Geometry check sheet. Reference: the model listing, model coordinates, mm. Face numbers are marked on the shaded views. A direction names the side the tool comes from. Give positions to 0.01 mm unless a question says otherwise; leave off trailing zeros. Order: outer loops, then holes, each group sorted by start corner. A loop starts at its lowest first (then second) coordinate and runs counter-clockwise, first axis right, second up. Notation, with made-up numbers: M 21,-24.75 L 64,-24.75 A15 ccw 64,-11.75 Z; hole C 33,-8.75 d5. An arc over 180 degrees is marked long. One line per question, with ' | ' between items. Start each with the question number.
from build123d import *

# Parameters (mm, degrees)
SKETCH1_R           = 15
BOSS_EXTRUDE2_DEPTH = 60


with BuildPart() as part:
    # Sketch1 → Boss-Extrude2 (new body)
    # profile 1 of 2: a face of its own
    with BuildSketch(Plane.XY):
        with BuildLine():
            Line((-12.60240546, 38.711870299), (-12.60240546, -11.288129701))
            Line((-12.60240546, -11.288129701), (47.39759454, -11.288129701))
            Line((47.39759454, -11.288129701), (47.39759454, 38.711870299))
            ThreePointArc((47.39759454, 38.711870299), (17.39759454, 68.711870299), (-12.60240546, 38.711870299))
        make_face()
        with Locations((17.39759454, 38.711870299)):
            Circle(SKETCH1_R, mode=Mode.SUBTRACT)
    # profile 2 of 2: a face of its own
    with BuildSketch(Plane.XY):
        Polygon((-42.60240546, -11.288129701), (77.39759454, -11.288129701), (77.39759454, -36.288129701), (62.39759454, -36.288129701), (62.39759454, -21.288129701), (-27.60240546, -21.288129701), (-27.60240546, -36.288129701), (-42.60240546, -36.288129701), align=None)
    extrude(amount=BOSS_EXTRUDE2_DEPTH)


solid = part.part
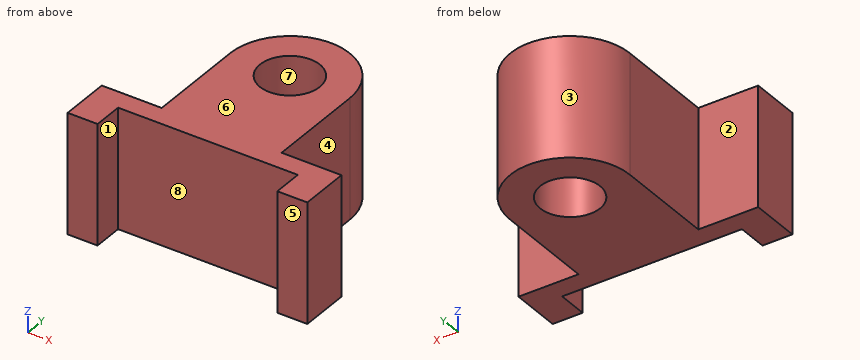
Item 1: Cross-section at C-C, the plane x = 4. Record the cut outline in (y, z).
Item 2: Depth check by flat-ended pin: pin 1 (25 mm diameter, centred on y = 20, z = 33, fed in from +X); pin 2 (18 mm diameter, centred on x = 4, z = 15.5, fed in from -Y); pin 3 (15 mm diameter, centred on y = 8, z = 20, fed in from -X); pin 4 (5 mm diameter, centred on x = 47.5, y = 18.5, fed in from +Z). Enter the tip coordinate at first touch or a pass-through.
Item 3: Cross-section at D-D, the plane x = -33. Record the cut outline in (y, z), plus the area to 3 significant figures.
Item 4: Material ranges on line 1 along X through (y, z) = (-32, 18.5); line 2 along Y through (x, z) = (70.5, 30); line 3 along Y through (x, z) = (-26.5, 45), recorded low to high.
Item 5: Cross-section at B-B, the plane z = 46.5. Record the cut outline in (x, y), plus the area to 3 significant figures.
Item 6: Set-up check for the marked faces 1, 2, 3, 4 and 5: record each of +Z, -Z, +X, -X, +Y, -Y from which the full face is reachable in a straight line by a thin tool's end or side.
Item 7: Cross-section at A-A, the plane y = -27.5. Record the cut outline in (x, z), plus the area to 3 significant figures.
Item 8: Mould release check, pull along Y, two halves, no side actions. Record for the marked faces 6, 7 and 8: released by +Y, released by -Y, zero draft, split by the parting line, or undercut.
Outcome:
1) outline: M -21.29,0 L 31.97,0 L 31.97,60 L -21.29,60 Z; M 45.46,0 L 65.55,0 L 65.55,60 L 45.46,60 Z
2) pin 1: stops at x = 47.4 | pin 2: stops at y = -21.29 | pin 3: stops at x = -12.6 | pin 4: stops at z = 60
3) outline: M -36.29,0 L -11.29,0 L -11.29,60 L -36.29,60 Z | area: 1,500 mm²
4) line 1: x = -42.6 to -27.6, 62.4 to 77.4 | line 2: y = -36.29 to -11.29 | line 3: y = -21.29 to -11.29
5) outline: M -42.6,-36.29 L -27.6,-36.29 L -27.6,-21.29 L 62.4,-21.29 L 62.4,-36.29 L 77.4,-36.29 L 77.4,-11.29 L 47.4,-11.29 L 47.4,38.71 A30 ccw -12.6,38.71 L -12.6,-11.29 L -42.6,-11.29 Z; hole C 17.4,38.71 d30 | area: 5,360 mm²
6) face 1: +Z, -Z, -Y | face 2: +Z, -Z, -X, +Y | face 3: +Z, -Z, +Y | face 4: +Z, -Z, +X, +Y | face 5: +Z, -Z, +X, -X, -Y
7) outline: M -42.6,0 L -27.6,0 L -27.6,60 L -42.6,60 Z; M 62.4,0 L 77.4,0 L 77.4,60 L 62.4,60 Z | area: 1,800 mm²
8) face 6: zero draft | face 7: undercut | face 8: released by -Y
